Can you work these out from the drawing? Everything is in mm from the part's minimum corner. A direction names the side the tool comes from. Give positions to 0.01 mm unless a question says otherwise; leave off trailing zeros. Order: outer loops, then holes, each group sorted by start corner. A loop starts at its lowest first (then second) coordinate and runs counter-clockwise, first axis right, second up. Notation, with made-up numbers: M -5.75,-18 L -0.75,-18 A14 cw -0.75,-9 Z; hole C 52.5,-9.5 d4. An arc over 180 degrees is marked long. Answer in a Markdown table with one row per item. Add a question column.
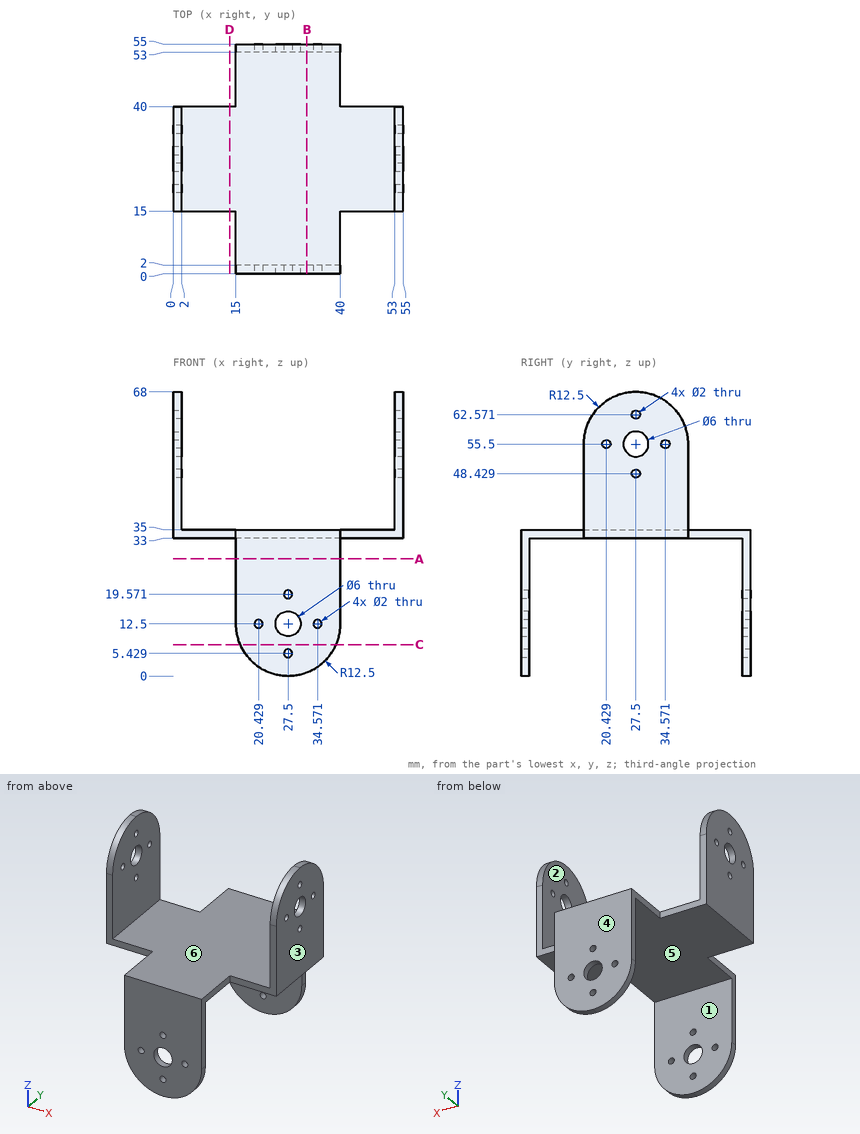
1. Suppose I cut it at A-A on z = 28. List the corners of the cut face in (x, y) for me.
2. Will these pins go through, and if not, where does the flat tip stop? P1, Ø4, axis at x = 30.5, y = 39, coming from the -Z side; P2, Ø5, axis at x = 43, y = 26, coming from the +Z side; P3, Ø16.5, axis at y = 4, z = 19, coming from the -X side.
3. Suppose I cut it at D-D on x = 13.5. List the corners of the cut face in (y, z) for me.
4. Suppose I cut it at B-B on x = 32. List the corners of the cut face in (y, z) for me, plus the area to 3 significant figures.
5. Suppose I cut it at C-C on z = 7.5. List the corners of the cut face in (x, y) for me.
6. If I drill on line 1 along Y through (x, z) = (33.5, 17); line 2 along Y through (x, z) = (53.8, 55.5), over which ranges is the centre line in solid material (lowest first)? Write a range as [from, to].
7. For the marked faces 4, 5 and 6, which set-ups out of +Z, -Z, +X, -X, +Y, -Y let a thin tool reach every point of the face, with its end or its side?
8. Thinking about a two-plate mould opening in X: for the marked faces 1, 2 and 3, which applies, pulls with the +X half, pulls with the -X half, needs draft (parallel to the pull), parting line crosses it, or undercut?
Findings below:
| question | item | result |
|---|---|---|
| 1 | outline | M 15,0 L 40,0 L 40,2 L 15,2 Z; M 15,53 L 40,53 L 40,55 L 15,55 Z |
| 2 | P1 | z = 33 |
| 2 | P2 | z = 35 |
| 2 | P3 | x = 15 |
| 3 | outline | M 15,33 L 40,33 L 40,35 L 15,35 Z |
| 4 | outline | M 0,0.84 L 2,0.84 L 2,33 L 53,33 L 53,0.84 L 55,0.84 L 55,35 L 0,35 Z |
| 4 | area | 239 mm2 |
| 5 | outline | M 16.04,0 L 38.96,0 L 38.96,2 L 16.04,2 Z; M 16.04,53 L 38.96,53 L 38.96,55 L 16.04,55 Z |
| 6 | line 1 | [0, 2], [53, 55] |
| 6 | line 2 | [15, 19.43], [21.43, 24.5], [30.5, 33.57], [35.57, 40] |
| 7 | face 4 | +Z, -Z, +X, -X, +Y |
| 7 | face 5 | -Z, +X, -X |
| 7 | face 6 | +Z, +Y, -Y |
| 8 | face 1 | needs draft |
| 8 | face 2 | undercut |
| 8 | face 3 | pulls with the +X half |
